Could you check a few things on this drawing? It's one solid part, dimensions in mm from its lowest x, y, z. A direction names the side the tool comes from. Round coordinates to 2 decimals unless told otherwise and drop trailing zeros. Write each loop counter-clockwise with the first axis right and the second up, starting at its lowest first coordinate (ties: lowest second). Pieces come first, ordered by that corner, then holes. Notation, with made-up numbers: (66, 0.5) -> (122, 0.5) arc R23 ccw to (122, 20.5) -> close; hole circle Ø4 at (41.25, 11). An arc over 180 degrees is marked (long way). Answer in a Markdown table with one row per item.
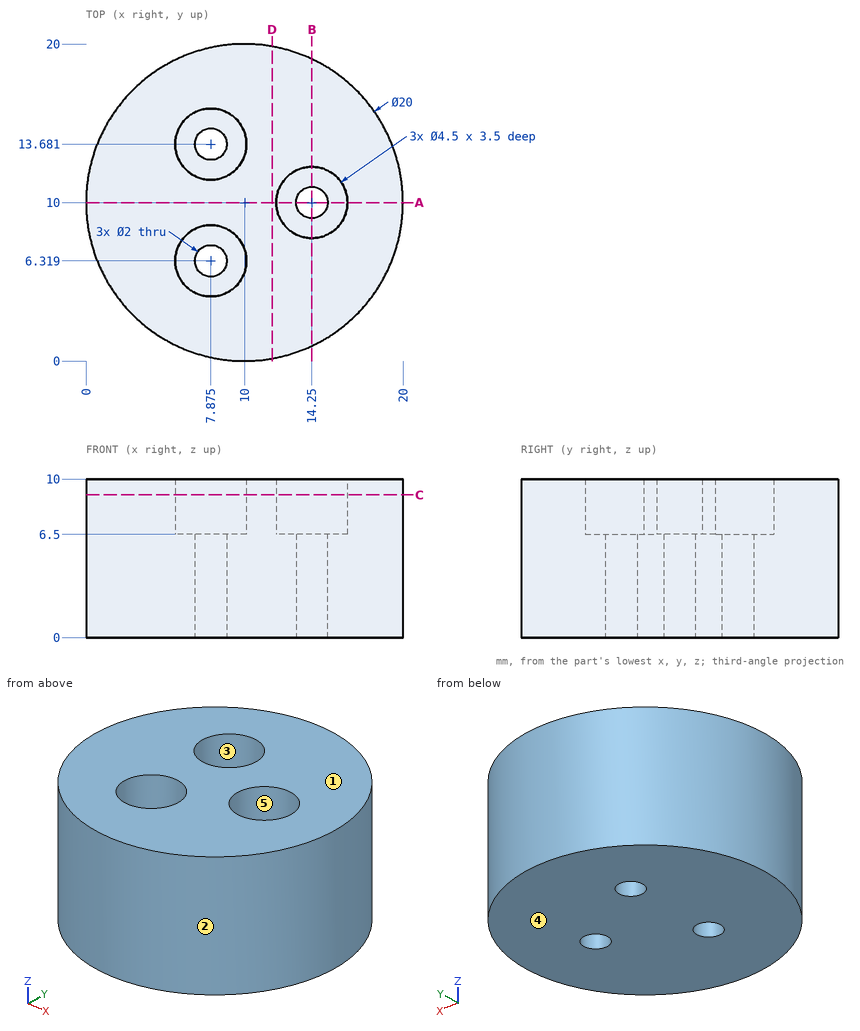
1) For pin 1 (5 mm diameter, centred on y = 2.5, z = 1.5, fed in from -X); pin 2 (6 mm diameter, centred on x = 14.25, y = 10, fed in from +Z); pin 3 (2 mm diameter, centred on x = 15.5, z = 7, fed in from +Y); pin 4 (2.5 mm diameter, centred on x = 14.25, y = 10, fed in from +Z), each with a flat end and sliding along its axis, tell me the tip position at first contact or that it passes through.
Response:
| item | result |
|---|---|
| pin 1 | stops at x = 1.34 |
| pin 2 | stops at z = 10 |
| pin 3 | stops at y = 18.93 |
| pin 4 | stops at z = 6.5 |
2) Which directions (+Z, -Z, +X, -X, +Y, -Y) give clear straight access to the entire face, cutting with the end or side of a thin tool? Please do the marked faces 4 and 5.
Response:
| item | result |
|---|---|
| face 4 | -Z, +X, -X, +Y, -Y |
| face 5 | +Z |
3) We'd pull the mould along Y, two halves only. Please class the marked faces 1, 2 and 3: +Y half, -Y half, draft (parallel to the pull), parting line (faces both ways), or undercut.
Response:
| item | result |
|---|---|
| face 1 | draft |
| face 2 | parting line |
| face 3 | undercut |
4) I need wall thicknesses on line 1 (Y direction, x = 6, z = 8) (1 decimal); line 2 (Y direction, x = 7.75, z = 2.5); line 3 (Y direction, x = 15.5, z = 7.5). Which ranges of each line are inside material? Lowest first, please. Write a range as [from, to].
Response:
| item | result |
|---|---|
| line 1 | y = [0.8, 5.1], [7.6, 12.4], [14.9, 19.2] |
| line 2 | y = [0.26, 5.33], [7.31, 12.69], [14.67, 19.74] |
| line 3 | y = [1.65, 8.13], [11.87, 18.35] |
5) I want a section at D-D, the plane x = 11.75. List the corners of the cut face in (y, z) for me (1 decimal), and give its area (3 significant figures).
Response:
| item | result |
|---|---|
| outline | (0.2, 0) -> (19.8, 0) -> (19.8, 10) -> (0.2, 10) -> close |
| area | 197 mm^2 |
6) I want a section at C-C, the plane z = 9. Count the separate pieces of the cut face and the enclosed holes in it.
Response:
| item | result |
|---|---|
| separate pieces | 1 |
| enclosed holes | 3 |
7) I want a section at A-A, the plane y = 10. List the corners of the cut face in (x, z) for me, and give its area (3 significant figures).
Response:
| item | result |
|---|---|
| outline | (0, 0) -> (13.25, 0) -> (13.25, 6.5) -> (12, 6.5) -> (12, 10) -> (0, 10) -> close; (15.25, 0) -> (20, 0) -> (20, 10) -> (16.5, 10) -> (16.5, 6.5) -> (15.25, 6.5) -> close |
| area | 171 mm^2 |
8) I want a section at B-B, the plane x = 14.25. List the corners of the cut face in (y, z) for me, and give its area (3 significant figures).
Response:
| item | result |
|---|---|
| outline | (0.95, 0) -> (9, 0) -> (9, 6.5) -> (7.75, 6.5) -> (7.75, 10) -> (0.95, 10) -> close; (11, 0) -> (19.05, 0) -> (19.05, 10) -> (12.25, 10) -> (12.25, 6.5) -> (11, 6.5) -> close |
| area | 152 mm^2 |
